Model file for the job. Use its own axes, mm. Face numbers are marked on the shaded views. Coordinates: 2 decimals unless noted, no trailing zeros. Loops run counter-clockwise (first coordinate to the right, second up) from the corner with the lowest first, then second, coordinate; pieces in that order, holes last. Notation, with made-up numbers: (47.5, 13) -> (53.5, 13) arc R35 ccw to (53.5, 45) -> close; hole circle Ø1 at (40.25, -7). An arc over 180 degrees is marked (long way). Use one line per item in the form item = value.
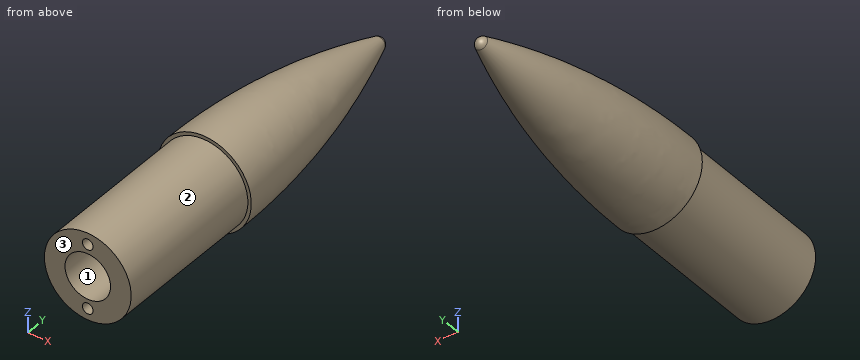
```python
from build123d import *

# Parameters (mm, degrees)
SKETCH2_R          = 2.35
CUT_EXTRUDE1_DEPTH = 10


with BuildPart() as part:
    # Sketch1 → Revolve3 (revolve)
    with BuildSketch(Plane.XY):
        with BuildLine():
            Line((-19.055, 0), (-20.555, 0))
            ThreePointArc((-20.555, 0), (-16.08987064, 51.964475913), (-2.825386961, 102.405506928))
            ThreePointArc((-2.825386961, 102.405506928), (-1.728341267, 103.849057861), (0, 104.396949286))
            Line((0, 104.396949286), (0, 102.396949286))
            Line((0, 102.396949286), (0, 71.445540784))
            Line((0, 71.445540784), (-10, 71.445540784))
            Line((-10, 71.445540784), (-10, -68.554459216))
            Line((-10, -68.554459216), (-17.055, -68.554459216))
            Line((-17.055, -68.554459216), (-19.055, -68.554459216))
            Line((-19.055, -68.554459216), (-19.055, 0))
        make_face()
    revolve(axis=Axis((0, 102.396949286, 0), (0, 1, 0)))

    # Sketch2 → Cut-Extrude1 (cut)
    with BuildSketch(Plane.XZ.offset(68.554459216)):
        with Locations((0, -14.055)):
            Circle(SKETCH2_R)
        with Locations((0, 14.055)):
            Circle(SKETCH2_R)
    extrude(amount=-CUT_EXTRUDE1_DEPTH, mode=Mode.SUBTRACT)


solid = part.part
```
Q1. Wall check: line 1 along Z through (x, y) = (0, -61.5) (3 decimals); line 2 along Z through (x, y) = (-3, 0.5); line 3 along X through (y, z) = (69.5, -6.5). Give the ranges that are in metal, low to high.
Result:
line_1 = -19.055 to -16.405, -11.705 to -10, 10 to 11.705, 16.405 to 19.055
line_2 = -20.33 to -9.54, 9.54 to 20.33
line_3 = -10.7 to -7.6, 7.6 to 10.7
Q2. Mould opens along X. For the marked faces 1, 2 and 3 say: released by +X, released by -X, zero draft, split by the parting line, or undercut.
Result:
face_1 = undercut
face_2 = split by the parting line
face_3 = zero draft
Q3. Pin check, flat tips, straight feed: pin 1 Ø5 at (x, z) = (-1, -14) entering from -Y; pin 2 Ø2 at (x, y) = (-12, 4) entering from -Z; pin 3 Ø1 at (x, y) = (3.5, -18) entering from -Z; pin 4 Ø4 at (y, z) = (49.5, 15.5) entering from -X. Stop position of each tip, or through.
Result:
pin_1 = -68.55
pin_2 = -17.33
pin_3 = -18.82
pin_4 = -9.55
Q4. Band-saw the part on A-A, the plane y = -10. Write the cut outline in (x, z) (3 decimals).
Result:
outline = circle Ø38.11 at (0, 0); hole circle Ø20 at (0, 0)
